Autodesk Fusion 360 part; units mm, degrees
sketch "Sketch1" plane through (0, 0, 0) normal (0, 0, 1) x (1, 0, 0)
  line L0 (0, 0) -> (17.6, 0)
  line L1 (17.6, 0) -> (17.6, 38)
  line L2 (17.6, 38) -> (0, 38)
  line L3 (0, 38) -> (0, 0)
  line L4 (-1.5, 0) -> (19.1, 0)
  line L5 (19.1, 0) -> (19.1, 39.5)
  line L6 (19.1, 39.5) -> (-1.5, 39.5)
  line L7 (-1.5, 39.5) -> (-1.5, 0)
  spline S0 degree 2 poles (0, 35.5) (2, 37) (8.8, 38) knots 0 0 0 0.926131 0.926131 0.926131 weights 1 3 1
  spline S1 degree 2 poles (17.6, 35.5) (15.497, 37.1201) (8.8, 38) knots 0 0 0 0.928188 0.928188 0.928188 weights 1 3 1
  dimension "d1" = 38
  dimension "d2" = 17.6
  dimension "d3" = 1.5
  dimension "d4" = 1.5
  dimension "d5" = 1.5
  dimension "d15" = 2.5
  dimension "d16" = 8.8
  dimension "d17" = 8.8
  dimension "d18" = 2.5
extrude "Extrude1" add sketch "Sketch1" along normal blind 1
extrude "Extrude2" add sketch "Sketch1" along normal blind 7.5 contours L1 L2 L3 L4 L5 L6 L7 | L2 L3 S0 | L1 L2 S1
fillet "Fillet1" radius 4.5 2 edges at (19.1, 39.5, 3.75) (-1.5, 39.5, 3.75)
Read the model definition and answer for the solid it produces. Units are mm, in the model's axes. Give positions to 0.01 mm unless a question says otherwise; leave off trailing zeros. Loops run counter-clockwise (first coordinate to the right, second up) from the corner with the lowest first, then second, coordinate; pieces in that order, holes last.
Item 1: This flat-tipped pin is pushed along its axis until it touches: pin 1 Ø1.5 at (x, y) = (4.5, 27) entering from +Z. Where does it stop, or does it pass through?
Item 2: Find the intervals of material crossed by line 1 along X through (y, z) = (6, 2.75); line 2 along Z through (x, y) = (16.75, 16.5); line 3 along Y through (x, z) = (9.25, 3), in increasing order.
Item 3: The part is cut by section A-A (y = 30). Write down the section's boundary in (x, z), and give its area (3 significant figures).
Taken from the geometry:
1. pin 1: stops at z = 1
2. line 1: x = -1.5 to 0, 17.6 to 19.1
2. line 2: z = 0 to 1
2. line 3: y = 37.94 to 39.5
3. outline: (-1.5, 0) - (19.1, 0) - (19.1, 7.5) - (17.6, 7.5) - (17.6, 1) - (0, 1) - (0, 7.5) - (-1.5, 7.5) - close
3. area: 40.1 mm2
